from build123d import *

# Parameters (mm, degrees)
F0_W     = 20
F0_H     = 40
F1_DEPTH = 5
F2_R     = 8.1
F3_DEPTH = 20
F5_DEPTH = 18
F6_R     = 1.65
F7_DEPTH = 29.699904
F8_R     = 2


with BuildPart() as f1:
    # F0 (on Top) → F1 (new body)
    with BuildSketch(Plane.XY):
        with Locations((-10, 20)):
            Rectangle(F0_W, F0_H)
    extrude(amount=F1_DEPTH)

    # F2 (on Right) → F3 (join)
    with BuildSketch(Plane.YZ):
        with BuildLine():
            ThreePointArc((7.556538, 17.198904), (20.056538, 4.698904), (32.556538, 17.198904))
            ThreePointArc((32.556538, 17.198904), (20.056538, 29.698904), (7.556538, 17.198904))
        make_face()
        with Locations((20.056538, 17.198904)):
            Circle(F2_R, mode=Mode.SUBTRACT)
        with BuildLine():
            Line((32.556538, 4.106051), (32.556538, 17.198904))
            ThreePointArc((32.556538, 17.198904), (20.056538, 4.698904), (7.556538, 17.198904))
            Line((7.556538, 17.198904), (7.556538, 4.106051))
            Line((7.556538, 4.106051), (32.340245, 4.106051))
            Line((32.340245, 4.106051), (32.556538, 4.106051))
        make_face()
    extrude(amount=-F3_DEPTH)

    # F4 (on face) → F5 (cut)
    with BuildSketch(Plane(origin=(-20, 0, 0), x_dir=(0, -1, 0), z_dir=(-1, 0, 0))):
        Polygon((-30.540984, 13.425348), (-22.030766, 6.232329), (-11.546319, 10.005885), (-9.572091, 20.97246), (-18.08231, 28.165478), (-28.566756, 24.391923), align=None)
    extrude(amount=-F5_DEPTH, mode=Mode.SUBTRACT)

    # F6 (on face) → F7 (cut, through all)
    with BuildSketch(Plane(origin=(0, 0, 0), x_dir=(1, 0, 0), z_dir=(0, 0, -1))):
        with Locations((-10, -4)):
            Circle(F6_R)
        with Locations((-10, -36)):
            Circle(F6_R)
    extrude(amount=-F7_DEPTH, mode=Mode.SUBTRACT)

    # F8
    f8_edges = [f1.edges().sort_by_distance(p)[0] for p in [
        (-20, 40, 2.5),
        (0, 40, 2.5),
        (0, 0, 2.5),
        (-20, 0, 2.5),
    ]]
    fillet(f8_edges, radius=F8_R)


solid = f1.part
Source: CAD feature listing. Evaluate the final solid. Frame: model axes, mm. A direction names the side the tool comes from. Give positions to 0.01 mm unless a question says otherwise; leave off trailing zeros. Loops run counter-clockwise (first coordinate to the right, second up) from the corner with the lowest first, then second, coordinate; pieces in that order, holes last. Notation, with made-up numbers: (-33.5, 48.25) -> (-20.5, 48.25) arc R28 ccw to (-20.5, 76.25) -> close; hole circle Ø3 at (89.5, -33). An arc over 180 degrees is marked (long way). Use a Markdown table: item, result. Add a question column.
1) Line query: line 1 along Y through (x, z) = (-10, 1.6); line 2 along X through (y, z) = (36, 2.4); line 3 along Z through (x, y) = (-13.75, 21). Output: solid intervals per line, ascending. Write a range as [from, to].
2) Section query A-A, the plane x = -10. Return the cut outline in (y, z).
3) Section query D-D, the plane z = 2.5. Return the cut outline in (x, y), then the cut area to 3 significant figures.
4) Section query C-C, the plane x = -14. Return the cut outline in (y, z), then the cut area to 3 significant figures.
5) Section query B-B, the plane y = 4. Return the cut outline in (x, z).
6) Reachability of faces 4 (the face through (-11.126, 16.862, 8.093)), 5 (the face through (-10, 40, 2)), 6 (the face through (-10, 2, 5)) from +Z, -Z, +X, -X, +Y, -Y: full face, straight path, thin tool, end or side. Return the list, or none.
7) Pull-direction query (Z, two-part tool) for faces 1 (the face through (-10, 38, 5)), 2 (the face through (-9.11, 34.61, 2.46)), 3 (the face through (-0.986, 14.087, 22.673)); classes: +Z half, -Z half, draft (parallel to the pull), parting line (faces both ways), or undercut.
8) First-contact query: pin 1 (2.5 mm diameter, centred on x = -14.5, y = 5, fed in from +Z); pin 2 (10 mm diameter, centred on x = -10, y = 11, fed in from +Z); pin 3 (5 mm diameter, centred on x = -10.5, z = 11.5, fed in from -Y). Flat tips, straight axial feed; report the tip coordinate or a pass-through.
Numbers:
| question | item | result |
|---|---|---|
| 1 | line 1 | y = [0, 2.35], [5.65, 34.35], [37.65, 40] |
| 1 | line 2 | x = [-20, -11.65], [-8.35, 0] |
| 1 | line 3 | z = [0, 6.6], [27.12, 29.66] |
| 2 | outline | (0, 0) -> (2.35, 0) -> (2.35, 5) -> (0, 5) -> close; (5.65, 0) -> (34.35, 0) -> (34.35, 5) -> (32.56, 5) -> (32.56, 17.2) arc R12.5 ccw to (7.56, 17.2) -> (7.56, 5) -> (5.65, 5) -> close; (37.65, 0) -> (40, 0) -> (40, 5) -> (37.65, 5) -> close; hole (9.57, 20.97) -> (11.55, 10.01) -> (22.03, 6.23) -> (30.54, 13.43) -> (28.57, 24.39) -> (18.08, 28.17) -> close |
| 3 | outline | (-20, 2) arc R2 ccw to (-18, 0) -> (-2, 0) arc R2 ccw to (0, 2) -> (0, 38) arc R2 ccw to (-2, 40) -> (-18, 40) arc R2 ccw to (-20, 38) -> close; hole circle Ø3.3 at (-10, 4); hole circle Ø3.3 at (-10, 36) |
| 3 | area | 779 mm2 |
| 4 | outline | (0, 0) -> (40, 0) -> (40, 5) -> (32.56, 5) -> (32.56, 17.2) arc R12.5 ccw to (7.56, 17.2) -> (7.56, 5) -> (0, 5) -> close; hole (9.57, 20.97) -> (11.55, 10.01) -> (22.03, 6.23) -> (30.54, 13.43) -> (28.57, 24.39) -> (18.08, 28.17) -> close |
| 4 | area | 428 mm2 |
| 5 | outline | (-20, 0) -> (-11.65, 0) -> (-11.65, 5) -> (-20, 5) -> close; (-8.35, 0) -> (0, 0) -> (0, 5) -> (-8.35, 5) -> close |
| 6 | face 4 | -X |
| 6 | face 5 | +Z, -Z, +X, -X, +Y |
| 6 | face 6 | +Z, +X, -X, -Y |
| 7 | face 1 | +Z half |
| 7 | face 2 | draft |
| 7 | face 3 | undercut |
| 8 | pin 1 | stops at z = 5 |
| 8 | pin 2 | stops at z = 29.02 |
| 8 | pin 3 | stops at y = 7.56 |
